Geometry check sheet. Reference: the model listing, model coordinates, mm. Face numbers are marked on the shaded views. A direction names the side the tool comes from. Coordinates: 2 decimals unless noted, no trailing zeros. Loops run counter-clockwise (first coordinate to the right, second up) from the corner with the lowest first, then second, coordinate; pieces in that order, holes last. Notation, with made-up numbers: (33, -35) - (45, -35) arc R19 cw to (45, -7) - close; hole circle Ø6 at (-32, -3.5). An arc over 180 degrees is marked (long way). Write each question's results on one line, items separated by ' | '. Start each with the question number.
(1) Sectioned sample at B-B (y = -6.5). Enter the section's corners in (x, z).
(2) Sectioned sample at D-D (x = 19). Enter the section's corners in (y, z), plus the area to 3 significant figures.
(3) Mould release check, pull along X, two halves, no side actions. Record for the marked faces 1, 2, 3 and 4: pulls with the +X half, pulls with the -X half, needs draft (parallel to the pull), parting line crosses it, or undercut.
(4) Access from +Z, -Z, +X, -X, +Y, -Y to the whole of each face (thin tool, end or side, straight path). Record for the marked faces 5, 6, 7, 8 and 9.
(5) Sectioned sample at A-A (z = 11.5). Enter the section's corners in (x, y), plus the area to 3 significant figures.
(6) Go/stop test with flat-tipped pins: pin 1 Ø1 at (y, z) = (6.5, 16) entering from -X; pin 2 Ø12 at (y, z) = (2.5, 19) entering from +X; pin 3 Ø13 at (x, y) = (-19, -4.5) entering from +Z. Record where each tip stops, or that it passes through.
(7) Sectioned sample at C-C (y = -2.5). Enter the section's corners in (x, z).
(8) Material ranges on probe 1 along Y at (x, z) = (19, 2.8); probe 2 along Y at (x, z) = (3, 3.5); probe 3 along X at (y, z) = (-7.5, 4), recorded low to high.
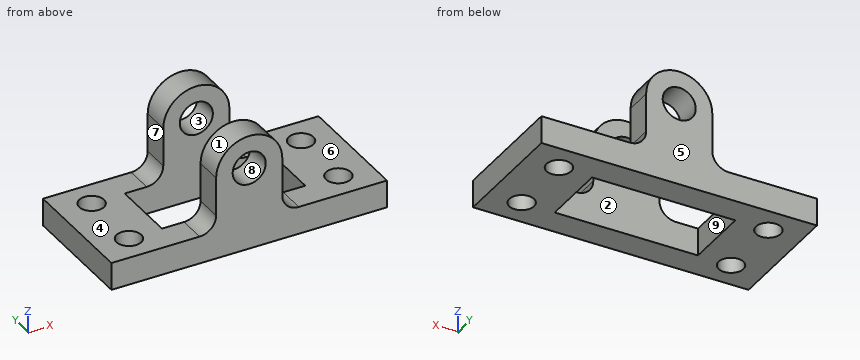
from build123d import *

# Parameters (mm, degrees)
SKETCH_1_W                = 6
SKETCH_1_H                = 5
REVOLVE_1_ANGLE           = 180
SKETCH_2_W                = 12
SKETCH_2_H                = 5
EXTRUDE_1_DEPTH           = 15
SKETCH_3_W                = 5
SKETCH_3_H                = 5
EXTRUDE_2_DEPTH           = 19
SKETCH_4_W                = 5
SKETCH_4_H                = 5
EXTRUDE_3_DEPTH           = 19
SKETCH_5_W                = 12
SKETCH_5_H                = 5
EXTRUDE_4_DEPTH           = 12
SKETCH_6_W                = 12
SKETCH_6_H                = 5
EXTRUDE_5_DEPTH           = 12
EXTRUDE_START             = 5
EXTRUDE_6_DEPTH           = 5
HOLE_WIZARD_6_0_6_1_D     = 6
HOLE_WIZARD_6_0_6_1_DEPTH = 5
HOLE_WIZARD_6_0_6_2_D     = 6
HOLE_WIZARD_6_0_6_2_DEPTH = 22
HOLE_WIZARD_4_5_4_5_1_D   = 4.5
FILLET_1_R                = 3


with BuildPart() as part:
    # 草图1 → 旋转1 (revolve)
    with BuildSketch(Plane(origin=(0, 0, 15), x_dir=(-1, 0, 0), z_dir=(0, 0, -1))):
        with Locations((3, -8.5)):
            Rectangle(SKETCH_1_W, SKETCH_1_H)
    revolve(axis=Axis((0, -6, 15), (0, 1, 0)), revolution_arc=REVOLVE_1_ANGLE)

    # 草图2 → 凸台-拉伸1 (add)
    with BuildSketch(Plane(origin=(0, 0, 15), x_dir=(-1, 0, 0), z_dir=(0, 0, -1))):
        with Locations((0, -8.5)):
            Rectangle(SKETCH_2_W, SKETCH_2_H)
    extrude(amount=EXTRUDE_1_DEPTH)

    # 草图3 → 凸台-拉伸2 (add)
    with BuildSketch(Plane.ZY.offset(6)):
        with Locations((2.5, -8.5)):
            Rectangle(SKETCH_3_W, SKETCH_3_H)
    extrude(amount=EXTRUDE_2_DEPTH)

    # 草图4 → 凸台-拉伸3 (add)
    with BuildSketch(Plane(origin=(6, 0, 0), x_dir=(0, 0, -1), z_dir=(1, 0, 0))):
        with Locations((-2.5, -8.5)):
            Rectangle(SKETCH_4_W, SKETCH_4_H)
    extrude(amount=EXTRUDE_3_DEPTH)

    # 草图5 → 凸台-拉伸4 (add)
    with BuildSketch(Plane(origin=(0, -6, 0), x_dir=(-1, 0, 0), z_dir=(0, 1, 0))):
        with Locations((-19, 2.5)):
            Rectangle(SKETCH_5_W, SKETCH_5_H)
    extrude(amount=EXTRUDE_4_DEPTH)

    # 草图6 → 凸台-拉伸5 (add)
    with BuildSketch(Plane(origin=(0, -6, 0), x_dir=(-1, 0, 0), z_dir=(0, 1, 0))):
        with Locations((19, 2.5)):
            Rectangle(SKETCH_6_W, SKETCH_6_H)
    extrude(amount=EXTRUDE_5_DEPTH)

    # 草图7 → 凸台-拉伸6 (add)
    with BuildSketch(Plane(origin=(0, 6, 0), x_dir=(-1, 0, 0), z_dir=(0, 1, 0)).offset(EXTRUDE_START)):
        with BuildLine():
            Line((25, 5), (25, 0))
            Line((25, 0), (-25, 0))
            Line((-25, 0), (-25, 5))
            Line((-25, 5), (-6, 5))
            Line((-6, 5), (-6, 15))
            ThreePointArc((-6, 15), (0, 21), (6, 15))
            Line((6, 15), (6, 5))
            Line((6, 5), (25, 5))
        make_face()
    extrude(amount=-EXTRUDE_6_DEPTH)

    # Ø6.0 (6) 直径孔1
    with Locations(Plane(origin=(0, 6, 0), x_dir=(-1, 0, 0), z_dir=(0, -1, 0))):
        with Locations((0, -15)):
            Hole(HOLE_WIZARD_6_0_6_1_D / 2, depth=HOLE_WIZARD_6_0_6_1_DEPTH)

    # Ø6.0 (6) 直径孔2
    with Locations(Plane(origin=(0, -11, 0), x_dir=(-1, 0, 0), z_dir=(0, -1, 0))):
        with Locations((0, -15)):
            Hole(HOLE_WIZARD_6_0_6_2_D / 2, depth=HOLE_WIZARD_6_0_6_2_DEPTH)

    # Ø4.5 (4.5) 直径孔1 (through all)
    with Locations(Plane(origin=(0, 0, 0), x_dir=(-1, 0, 0), z_dir=(0, 0, -1))):
        with Locations((-19, -6), (19, 6), (19, -6), (-19, 6)):
            Hole(HOLE_WIZARD_4_5_4_5_1_D / 2)

    # 圆角1
    fillet_1_edges = [part.edges().sort_by_distance(p)[0] for p in [
        (-6, -8.5, 5),
        (6, -8.5, 5),
        (-6, 8.5, 5),
        (6, 8.5, 5),
    ]]
    fillet(fillet_1_edges, radius=FILLET_1_R)


solid = part.part
Outcome:
1) outline: (-25, 0) - (-21.19, 0) - (-21.19, 5) - (-25, 5) - close; (-16.81, 0) - (16.81, 0) - (16.81, 5) - (9, 5) arc R3 cw to (6, 8) - (6, 15) arc R6 ccw to (-6, 15) - (-6, 8) arc R3 cw to (-9, 5) - (-16.81, 5) - close; (21.19, 0) - (25, 0) - (25, 5) - (21.19, 5) - close; hole circle Ø6 at (0, 15)
2) outline: (-11, 0) - (-8.25, 0) - (-8.25, 5) - (-11, 5) - close; (-3.75, 0) - (3.75, 0) - (3.75, 5) - (-3.75, 5) - close; (8.25, 0) - (11, 0) - (11, 5) - (8.25, 5) - close | area: 65.0 mm2
3) face 1: parting line crosses it | face 2: undercut | face 3: undercut | face 4: needs draft
4) face 5: +Z, -Z, +X, -X, +Y | face 6: +Z, +X, +Y, -Y | face 7: +Z, -X, +Y, -Y | face 8: +Y, -Y | face 9: +Z, -Z
5) outline: (-6, -11) - (6, -11) - (6, -6) - (-6, -6) - close; (-6, 6) - (6, 6) - (6, 11) - (-6, 11) - close | area: 120 mm2
6) pin 1: stops at x = -5.98 | pin 2: stops at x = 6 | pin 3: stops at z = 5
7) outline: (-25, 0) - (-13, 0) - (-13, 5) - (-25, 5) - close; (13, 0) - (25, 0) - (25, 5) - (13, 5) - close
8) probe 1: y = -11 to -8.25, -3.75 to 3.75, 8.25 to 11 | probe 2: y = -11 to -6, 6 to 11 | probe 3: x = -25 to -20.68, -17.32 to 17.32, 20.68 to 25
